from build123d import *

# Parameters (mm, degrees)
SKETCH_1_W                   = 40
SKETCH_1_H                   = 20
EXTRUDE_1_DEPTH              = 39
CHAMFER_1_SIZE               = 1
SKETCH_12_W                  = 18
SKETCH_12_H                  = 4
EXTRUDE_7_DEPTH              = 8
SKETCH_13_R                  = 2
CUT_EXTRUDE_2_DEPTH          = 43.95346319
FILLET_3_R                   = 1
SKETCH_14_R                  = 6
EXTRUDE_8_DEPTH              = 1
SKETCH_15_R                  = 5
EXTRUDE_9_DEPTH              = 1
SKETCH_16_R                  = 3
EXTRUDE_10_DEPTH             = 4
HOLE_WIZARD_M3_2_D           = 2.5
HOLE_WIZARD_M3_2_DEPTH       = 7.5
HOLE_WIZARD_M3_2_CSINK_D     = 3.05
HOLE_WIZARD_M3_2_CSINK_ANGLE = 90
HOLE_WIZARD_M3_2_TIP         = 0.751075774
CHAMFER_3_SIZE               = 1


with BuildPart() as part:
    # 草图1 → 凸台-拉伸1 (new body)
    with BuildSketch(Plane(origin=(0, 0, 0), x_dir=(1, 0, 0), z_dir=(0, 1, 0))):
        Rectangle(SKETCH_1_W, SKETCH_1_H)
    extrude(amount=EXTRUDE_1_DEPTH)

    # 倒角1
    chamfer_1_edges = [part.edges().sort_by_distance(p)[0] for p in [
        (-20, 39, 0),
        (0, 39, 10),
        (20, 39, 0),
        (0, 0, 10),
        (-20, 0, 0),
        (0, 0, -10),
        (20, 0, 0),
        (20, 19.5, 10),
        (-20, 19.5, 10),
        (-20, 19.5, -10),
        (20, 19.5, -10),
        (0, 39, -10),
    ]]
    chamfer(chamfer_1_edges, length=CHAMFER_1_SIZE)

    # 草图12 → 凸台-拉伸7 (add)
    with BuildSketch(Plane.ZY.offset(20)):
        with Locations((0, 29)):
            Rectangle(SKETCH_12_W, SKETCH_12_H)
    extrude_7 = extrude(amount=EXTRUDE_7_DEPTH)

    # 镜向1: 凸台-拉伸7 across plane
    add(extrude_7.mirror(Plane(origin=(0, 0, 0), x_dir=(0, 0, 1), z_dir=(1, 0, 0))))

    # 草图13 → 切除-拉伸2 (cut, through all)
    with BuildSketch(Plane(origin=(0, 31, 0), x_dir=(1, 0, 0), z_dir=(0, 1, 0))):
        with Locations(Location((-24, 5, 0), (0, 0, 270))):
            Circle(SKETCH_13_R)
        with Locations(Location((-24, -5, 0), (0, 0, 270))):
            Circle(SKETCH_13_R)
        with Locations(Location((24, -5, 0), (0, 0, 270))):
            Circle(SKETCH_13_R)
        with Locations(Location((24, 5, 0), (0, 0, 90))):
            Circle(SKETCH_13_R)
    extrude(amount=-CUT_EXTRUDE_2_DEPTH, mode=Mode.SUBTRACT)

    # 圆角3
    fillet_3_edges = [part.edges().sort_by_distance(p)[0] for p in [
        (-28, 29, 9),
        (-28, 29, -9),
        (28, 29, 9),
        (28, 29, -9),
    ]]
    fillet(fillet_3_edges, radius=FILLET_3_R)

    # 草图14 → 凸台-拉伸8 (add)
    with BuildSketch(Plane(origin=(0, 39, 0), x_dir=(1, 0, 0), z_dir=(0, 1, 0))):
        with Locations(Location((-10, 0, 0), (0, 0, 90))):
            Circle(SKETCH_14_R)
    extrude(amount=EXTRUDE_8_DEPTH)

    # 草图15 → 凸台-拉伸9 (add)
    with BuildSketch(Plane(origin=(0, 40, 0), x_dir=(1, 0, 0), z_dir=(0, 1, 0))):
        with Locations(Location((-10, 0, 0), (0, 0, 270))):
            Circle(SKETCH_15_R)
    extrude(amount=EXTRUDE_9_DEPTH)

    # 草图16 → 凸台-拉伸10 (add)
    with BuildSketch(Plane(origin=(0, 41, 0), x_dir=(1, 0, 0), z_dir=(0, 1, 0))):
        with Locations(Location((-10, 0, 0), (0, 0, 270))):
            Circle(SKETCH_16_R)
    extrude(amount=EXTRUDE_10_DEPTH)

    # M3 螺纹孔2
    with Locations(Plane(origin=(0, 45, 0), x_dir=(1, 0, 0), z_dir=(0, 1, 0))):
        with Locations((-10, 0)):
            CounterSinkHole(HOLE_WIZARD_M3_2_D / 2, HOLE_WIZARD_M3_2_CSINK_D / 2, depth=HOLE_WIZARD_M3_2_DEPTH, counter_sink_angle=HOLE_WIZARD_M3_2_CSINK_ANGLE)
            with Locations((0, 0, -(HOLE_WIZARD_M3_2_DEPTH + HOLE_WIZARD_M3_2_TIP / 2))):  # 118° drill point
                Cone(0, HOLE_WIZARD_M3_2_D / 2, HOLE_WIZARD_M3_2_TIP, mode=Mode.SUBTRACT)

    # 倒角3
    chamfer_3_edges = [part.edges().sort_by_distance(p)[0] for p in [
        (-10, 41, -5),
    ]]
    chamfer(chamfer_3_edges, length=CHAMFER_3_SIZE - 0.0001)  # a hair under: the kernel refuses the full size


solid = part.part
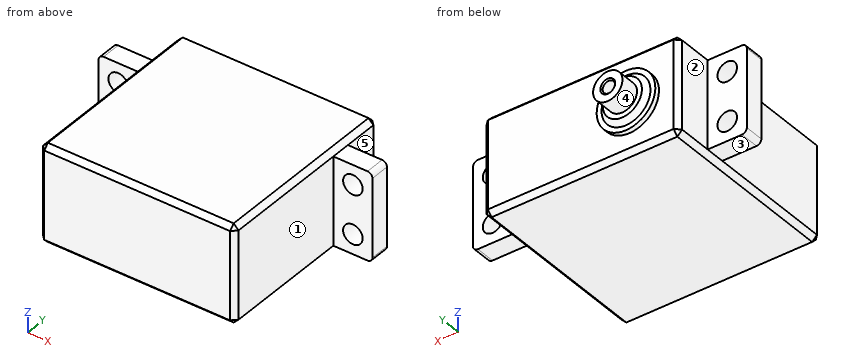
Work out the finished part from the listing and answer in its coordinate system (mm). Face numbers are marked on the shaded views. A direction names the side the tool comes from. Give positions to 0.01 mm unless a question says otherwise; leave off trailing zeros. Order: outer loops, then holes, each group sorted by start corner. A loop starts at its lowest first (then second) coordinate and runs counter-clockwise, first axis right, second up. Notation, with made-up numbers: (-36, -2) - (-10, -2) arc R25 cw to (-10, 26) - close; hole circle Ø5 at (3, -30.75). An arc over 180 degrees is marked (long way). Answer as CSV lines item,"result". Start each with the question number.
Q1. Find the intervals of material crossed by L1, parallel to X at y = 29.1, z = -5; L2, parallel to Y at x = -1, z = -4.5; L3, parallel to X at y = 5, z = 5.25, in increasing order. Write a range as [from, to].
Q2. Given pin 1 Ø3 at (x, z) = (-10, 0) entering from -Y; pin 2 Ø4 at (x, z) = (-26, 2) entering from +Y; pin 3 Ø1.2 at (x, y) = (-25, 29.5) entering from +Z; pin 4 Ø1.2 at (x, y) = (23, 28) entering from -Z, each flat-ended and moving along its own axis, determine where each tip first touches the part or whether it passes through.
Q3. The part is cut by section A-A (x = 24). Write down the section's boundary in (y, z).
Q4. For the marked faces 1, 2, 3, 4 and 5, determine the directions among +Z, -Z, +X, -X, +Y, -Y from which every point of the face is accessible in a straight line to the end or side of a thin tool.
Q5. The part is cut by section C-C (x = 14). Write down the section's boundary in (y, z), then the cut area to 3 significant figures.
Q6. The part is cut by section B-B (y = 6). Write down the section's boundary in (x, z).
Check result:
1,L1,"x = [-28, -26], [-22, 22], [26, 28]"
1,L2,"y = [0, 39]"
1,L3,"x = [-20, 20]"
2,pin 1,"stops at y = 0"
2,pin 2,"stops at y = 31"
2,pin 3,"stops at z = 9"
2,pin 4,"stops at z = -9"
3,outline,"(27, -9) - (31, -9) - (31, -7) - (27, -7) - close; (27, -3) - (31, -3) - (31, 3) - (27, 3) - close; (27, 7) - (31, 7) - (31, 9) - (27, 9) - close"
4,face 1,"+Z, -Z, +X, -Y"
4,face 2,"+Z, -Z, -X, +Y"
4,face 3,"-Z, -X, +Y, -Y"
4,face 4,"+Y"
4,face 5,"+Z, -Z, +X, +Y"
5,outline,"(0, -9) - (1, -10) - (38, -10) - (39, -9) - (39, 9) - (38, 10) - (1, 10) - (0, 9) - close"
5,area,"778 mm²"
6,outline,"(-20, -9) - (-19, -10) - (19, -10) - (20, -9) - (20, 9) - (19, 10) - (-19, 10) - (-20, 9) - close"
